from build123d import *

# Parameters (mm, degrees)
SKETCH2_W           = 1.75
SKETCH2_H           = 1.43
BOSS_EXTRUDE1_DEPTH = 1.4
SKETCH3_R           = 10.06
CUT_EXTRUDE1_DEPTH  = 21.193741605


with BuildPart() as part:
    # Sketch1 → Revolve1 (revolve)
    with BuildSketch(Plane.XY, mode=Mode.PRIVATE) as revolve1_sk:
        Polygon((0, 0), (0, 24.17), (3.25, 24.17), (3.25, 19.49), (3.39, 19.49), (3.39, 15.87), (4.2, 15.87), (4.2, 8.17), (7.56, 8.17), (7.56, 10.57), (9.56, 10.57), (9.56, 4.04), (7.56, 4.04), (7.56, 6.89), (3.365, 6.89), (3.365, 2.46), (2, 2.46), (2, 0), align=None)
    revolve(revolve1_sk.sketch.rotate(Axis((0, 0, 0), (0, 1, 0)), 90), axis=Axis((0, 0, 0), (0, 1, 0)))

    # Sketch2 → Boss-Extrude1 (add)
    with BuildSketch(Plane(origin=(0, 24.17, 0), x_dir=(1, 0, 0), z_dir=(0, 1, 0))):
        with Locations((0, 2.115)):
            Rectangle(SKETCH2_W, SKETCH2_H)
    extrude(amount=BOSS_EXTRUDE1_DEPTH)

    # Sketch3 → Cut-Extrude1 (cut, through all)
    with BuildSketch(Plane(origin=(0, 10.57, 0), x_dir=(1, 0, 0), z_dir=(0, 1, 0))):
        Circle(SKETCH3_R)
        Polygon((0, 9.56), (-0.891981902, 8.201638147), (-2.055117408, 9.336492513), (-2.634237624, 7.818138662), (-4.014139811, 8.676421012), (-4.253319322, 7.069071703), (-5.785465497, 7.610649708), (-5.673520536, 5.989462808), (-7.286269247, 6.189012883), (-6.828434235, 4.629793289), (-8.446375145, 4.477984693), (-7.664057938, 3.053639782), (-9.211537928, 2.557570916), (-8.141318811, 1.334701472), (-9.545979436, 0.517567966), (-8.237900664, -0.446645996), (-9.434061555, -1.546635887), (-7.949287438, -2.207108793), (-8.881017441, -3.538520765), (-7.288974367, -3.864369636), (-7.912706822, -5.364948345), (-6.287836955, -5.340936849), (-6.574406827, -6.940516903), (-4.992687275, -6.567767792), (-4.928694875, -8.191554604), (-3.464085088, -7.487497212), (-3.052522628, -9.059564317), (-1.773506132, -8.057119585), (-1.033617816, -9.50395887), (0, -8.25), (1.033617816, -9.50395887), (1.773506132, -8.057119585), (3.052522628, -9.059564317), (3.464085088, -7.487497212), (4.928694875, -8.191554604), (4.992687275, -6.567767792), (6.574406827, -6.940516903), (6.287836955, -5.340936849), (7.912706822, -5.364948345), (7.288974367, -3.864369636), (8.881017441, -3.538520765), (7.949287438, -2.207108793), (9.434061555, -1.546635887), (8.237900664, -0.446645996), (9.545979436, 0.517567966), (8.141318811, 1.334701472), (9.211537928, 2.557570916), (7.664057938, 3.053639782), (8.446375145, 4.477984693), (6.828434235, 4.629793289), (7.286269247, 6.189012883), (5.673520536, 5.989462808), (5.785465497, 7.610649708), (4.253319322, 7.069071703), (4.014139811, 8.676421012), (2.634237624, 7.818138662), (2.055117408, 9.336492513), (0.891981902, 8.201638147), align=None, mode=Mode.SUBTRACT)
    extrude(amount=-CUT_EXTRUDE1_DEPTH, mode=Mode.SUBTRACT)


solid = part.part
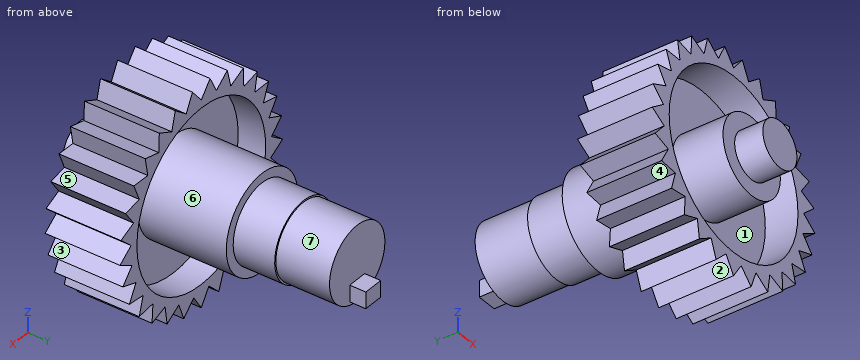
Read the model definition and answer for the solid it produces. Units are mm, in the model's axes. Face numbers are marked on the shaded views. A direction names the side the tool comes from. Coordinates: 2 decimals unless noted, no trailing zeros. Order: outer loops, then holes, each group sorted by start corner. A loop starts at its lowest first (then second) coordinate and runs counter-clockwise, first axis right, second up. Notation, with made-up numbers: M 14.5,-8.5 L 31.5,-8.5 A25 ccw 31.5,12.5 Z; hole C -39,44.25 d4. An arc over 180 degrees is marked long. Put each result on its own line as item: value. Start each with the question number.
Item 1: Section B-B, the plane z = 2.75 is taken. Determine the outline of the cut face in (x, y), plus the area to 3 significant figures.
Item 2: For the marked faces 1, 2, 3 and 4, determine the directions among +Z, -Z, +X, -X, +Y, -Y from which every point of the face is accessible in a straight line to the end or side of a thin tool.
Item 3: Section D-D, the plane z = -5 is taken. Determine the outline of the cut face in (x, y).
Item 4: Given pin 1 Ø6 at (y, z) = (17.5, -2) entering from +X; pin 2 Ø1 at (y, z) = (8.5, 5.5) entering from -X; pin 3 Ø1.5 at (x, z) = (6, -5.5) entering from -Y; pin 4 Ø5 at (y, z) = (22.5, 6.5) entering from -X, each flat-ended and moving along its own axis, determine where each tip first touches the part or whether it passes through.
Item 5: Section C-C, the plane y = 11.5 is taken. Determine the outline of the cut face in (x, z), plus the area to 3 significant figures.
Item 6: The mould has two halves that part along X. Classify the marked faces 5, 6 and 7: +X half, -X half, draft (parallel to the pull), parting line (faces both ways), or undercut.
Item 7: Consider probe 1 along X at (y, z) = (10.05, 0); probe 2 along X at (y, z) = (5.4, 0) (3 decimals); probe 3 along Y at (x, z) = (1.25, -1). Determine where each line is inside the solid, lowest interval first. Write a range as [from, to].
Item 8: Section A-A, the plane z = 8.75 is taken. Determine the outline of the cut face in (x, y), plus the area to 3 significant figures.
Computed:
1. outline: M -8.33,4.04 L -7.04,4.04 L -7.04,6.89 L -1.94,6.89 L -1.94,2.46 L 1.94,2.46 L 1.94,6.89 L 7.04,6.89 L 7.04,4.04 L 8.33,4.04 L 8.33,10.57 L 7.04,10.57 L 7.04,8.17 L 3.17,8.17 L 3.17,15.87 L 1.98,15.87 L 1.98,19.49 L 1.73,19.49 L 1.73,24.17 L -1.73,24.17 L -1.73,19.49 L -1.98,19.49 L -1.98,15.87 L -3.17,15.87 L -3.17,8.17 L -7.04,8.17 L -7.04,10.57 L -8.33,10.57 Z
1. area: 131 mm2
2. face 1: -Y
2. face 2: -Z, +Y, -Y
2. face 3: +X, +Y, -Y
2. face 4: -X, +Y, -Y
3. outline: M -6.94,4.04 L -5.67,4.04 L -5.67,6.89 L 5.67,6.89 L 5.67,4.04 L 6.94,4.04 L 6.94,10.57 L 5.67,10.57 L 5.67,8.17 L -5.67,8.17 L -5.67,10.57 L -6.94,10.57 Z
4. pin 1: stops at x = 4.2
4. pin 2: stops at x = -7.91
4. pin 3: stops at y = 4.04
4. pin 4: passes through
5. outline: C 0,0 d8.4
5. area: 55.4 mm2
6. face 5: +X half
6. face 6: undercut
6. face 7: parting line
7. probe 1: x = [-8.84, -7.56], [-4.2, 4.2], [7.56, 8.84]
7. probe 2: x = [-8.844, -7.56], [-3.365, 3.365], [7.56, 8.844]
7. probe 3: y = [0, 24.17]
8. outline: M -3.13,4.04 L -2.66,4.04 L -2.66,10.57 L -3.13,10.57 Z; M -1.42,4.04 L -0.41,4.04 L -0.41,10.57 L -1.42,10.57 Z; M 0.41,4.04 L 1.42,4.04 L 1.42,10.57 L 0.41,10.57 Z; M 2.66,4.04 L 3.13,4.04 L 3.13,10.57 L 2.66,10.57 Z
8. area: 19.4 mm2
